```python
from build123d import *

# Parameters (mm, degrees)
F0_W     = 10.66
F0_H     = 5
F1_DEPTH = 8.5
F2_W     = 1.5
F2_H     = 1.5
F3_DEPTH = 7
F4_W     = 0.6
F4_H     = 0.4
F5_DEPTH = 3


with BuildPart() as f1:
    # F0 (on Top) → F1 (new body)
    with BuildSketch(Plane.XY):
        Rectangle(F0_W, F0_H)
    extrude(amount=F1_DEPTH)

    # F2 (on face) → F3 (cut)
    with BuildSketch(Plane.XY.offset(8.5)):
        with Locations((-3.81, 1.27)):
            Rectangle(F2_W, F2_H)
        with Locations((-3.81, -1.27)):
            Rectangle(F2_W, F2_H)
        with Locations((-1.27, 1.27)):
            Rectangle(F2_W, F2_H)
        with Locations((-1.27, -1.27)):
            Rectangle(F2_W, F2_H)
        with Locations((1.27, 1.27)):
            Rectangle(F2_W, F2_H)
        with Locations((1.27, -1.27)):
            Rectangle(F2_W, F2_H)
        with Locations((3.81, 1.27)):
            Rectangle(F2_W, F2_H)
        with Locations((3.81, -1.27)):
            Rectangle(F2_W, F2_H)
        with Locations((6.35, 1.27)):
            Rectangle(F2_W, F2_H)
        with Locations((6.35, -1.27)):
            Rectangle(F2_W, F2_H)
        with Locations((8.89, 1.27)):
            Rectangle(F2_W, F2_H)
        with Locations((8.89, -1.27)):
            Rectangle(F2_W, F2_H)
    extrude(amount=-F3_DEPTH, mode=Mode.SUBTRACT)

    # F4 (on face) → F5 (join)
    with BuildSketch(Plane(origin=(0, 0, 0), x_dir=(1, 0, 0), z_dir=(0, 0, -1))):
        with Locations((-3.81, 1.27)):
            Rectangle(F4_W, F4_H)
        with Locations((-3.81, -1.27)):
            Rectangle(F4_W, F4_H)
        with Locations((-1.27, 1.27)):
            Rectangle(F4_W, F4_H)
        with Locations((-1.27, -1.27)):
            Rectangle(F4_W, F4_H)
        with Locations((1.27, 1.27)):
            Rectangle(F4_W, F4_H)
        with Locations((1.27, -1.27)):
            Rectangle(F4_W, F4_H)
        with Locations((3.81, 1.27)):
            Rectangle(F4_W, F4_H)
        with Locations((3.81, -1.27)):
            Rectangle(F4_W, F4_H)
    extrude(amount=F5_DEPTH)


with BuildPart() as f5:
    # F4 (on face) → F5, piece 2 (new body)
    with BuildSketch(Plane(origin=(0, 0, 0), x_dir=(1, 0, 0), z_dir=(0, 0, -1))):
        with Locations((6.35, 1.27)):
            Rectangle(F4_W, F4_H)
    extrude(amount=F5_DEPTH)


with BuildPart() as f5b:
    # F4 (on face) → F5, piece 3 (new body)
    with BuildSketch(Plane(origin=(0, 0, 0), x_dir=(1, 0, 0), z_dir=(0, 0, -1))):
        with Locations((6.35, -1.27)):
            Rectangle(F4_W, F4_H)
    extrude(amount=F5_DEPTH)


with BuildPart() as f5c:
    # F4 (on face) → F5, piece 4 (new body)
    with BuildSketch(Plane(origin=(0, 0, 0), x_dir=(1, 0, 0), z_dir=(0, 0, -1))):
        with Locations((8.89, 1.27)):
            Rectangle(F4_W, F4_H)
    extrude(amount=F5_DEPTH)


with BuildPart() as f5d:
    # F4 (on face) → F5, piece 5 (new body)
    with BuildSketch(Plane(origin=(0, 0, 0), x_dir=(1, 0, 0), z_dir=(0, 0, -1))):
        with Locations((8.89, -1.27)):
            Rectangle(F4_W, F4_H)
    extrude(amount=F5_DEPTH)


solid = f1.part
```
Part model, mm, in its own coordinate system. A direction names the side the tool comes from. Round coordinates to 2 decimals unless told otherwise and drop trailing zeros. Write each loop counter-clockwise with the first axis right and the second up, starting at its lowest first coordinate (ties: lowest second). Pieces come first, ordered by that corner, then holes.
Item 1: Which spindle directions (+Z, -Z, +X, -X, +Y, -Y) get a long thin tool onto all of the face, cutting with end or side? Do faces 4 (the flat face through (-4, 2.02, 5)), 5 (the flat face through (5.33, 0, 4)). Say none if no direction does.
Results:
face 4: +Z
face 5: +Z, -Z, +X, +Y, -Y
Item 2: Cut at B-B, the plane x = -1.75. Give the cut face in (y, z), plus the area to 3 significant figures.
Results:
outline: (-2.5, 0) - (2.5, 0) - (2.5, 8.5) - (2.02, 8.5) - (2.02, 1.5) - (0.52, 1.5) - (0.52, 8.5) - (-0.52, 8.5) - (-0.52, 1.5) - (-2.02, 1.5) - (-2.02, 8.5) - (-2.5, 8.5) - close
area: 21.5 mm2
Item 3: Probe L1, parallel to Y at x = 0.75, z = 2.25; L2, parallel to X at y = -0.7, z = 2; L3, parallel to Y at x = -1.25, z = -2.5. List the from-to ranges inside material, lowest first.
Results:
L1: y = -2.5 to -2.02, -0.52 to 0.52, 2.02 to 2.5
L2: x = -5.33 to -4.56, -3.06 to -2.02, -0.52 to 0.52, 2.02 to 3.06, 4.56 to 5.33
L3: y = -1.47 to -1.07, 1.07 to 1.47
Item 4: Cut at C-C, the plane y = -0.15. Give the cut face in (x, z).
Results:
outline: (-5.33, 0) - (5.33, 0) - (5.33, 8.5) - (-5.33, 8.5) - close
Item 5: Two-plate mould, pull along Y, no slides. Class faces 1 (the flat face through (0, 2.5, 4)), 2 (the flat face through (-5.33, 0, 4)), 3 (the flat face through (-1, 2.02, 5)): +Y half, -Y half, draft (parallel to the pull), parting line (faces both ways), or undercut.
Results:
face 1: +Y half
face 2: draft
face 3: undercut
Item 6: Cut at A-A, the plane z = -1. Count the separate pieces of the cut face and the enclosed holes in it, plus the area to 3 significant figures.
Results:
separate pieces: 8
enclosed holes: 0
area: 1.92 mm2
